Verification items for the finished model (mm, model axes). Face numbers are marked on the shaded views. A direction names the side the tool comes from. Give positions to 0.01 mm unless a question says otherwise; leave off trailing zeros. Write each loop counter-clockwise with the first axis right and the second up, starting at its lowest first coordinate (ties: lowest second). Pieces come first, ordered by that corner, then holes. Notation, with made-up numbers: (72.5, -17) -> (127.5, -17) arc R20 cw to (127.5, -8) -> close; hole circle Ø4 at (-6, -22.75). An arc over 180 degrees is marked (long way). Use CSV: the item, a comma, the result in double quotes. Start each with the question number.
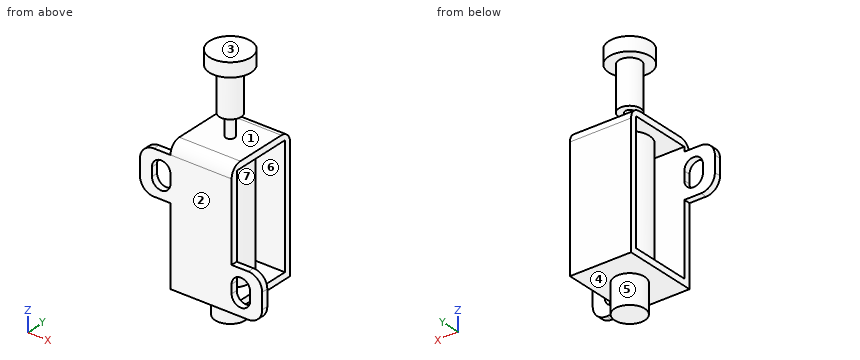
Autodesk Inventor part; units mm, degrees
ref_plane "Work Plane1" through (0, 8.5, 0) normal (0, 1, 0) x (1, 0, 0)
ref_plane "YZ Plane" through (0, 0, 0) normal (1, 0, 0) x (0, 1, 0)
ref_plane "XZ Plane" through (0, 0, 0) normal (0, 1, 0) x (-1, 0, 0)
sketch "Sketch1" plane through (0, 0, 0) normal (0, 1, 0) x (-1, 0, 0)
  line L0 (7, 15.2) -> (-7, 15.2)
  line L1 (-7, 15.2) -> (-7, -15.2)
  line L2 (-7, -15.2) -> (7, -15.2)
  line L3 (7, -15.2) -> (7, 15.2)
  point P0 (0, 0)
  dimension "d0" = 30.4
  dimension "d1" = 14
  dimension "d2" = 7
  dimension "d3" = 15.2
extrude "Extrusion1" add sketch "Sketch1" along normal blind 17
fillet "Fillet1" radius 2.54 2 edges at (0, 17, 15.2) (0, 0, 15.2)
sketch "Sketch2" plane through (7, 0, -15.2) normal (1, 0, 0) x (0, 0, -1)
  line L0 (-1.5, 15.5) -> (-28.9, 15.5)
  line L1 (-28.9, 15.5) -> (-28.9, 1.5)
  line L2 (-28.9, 1.5) -> (-1.5, 1.5)
  line L3 (-1.5, 1.5) -> (-1.5, 15.5)
  line L4 (-28.9, 8.5) -> (-30.4, 8.5) construction
  line L5 (-30.4, 2.54) -> (-30.4, 14.46)
  line L6 (-1.5, 9.1916) -> (0, 9.1916) construction
  line L7 (0, 0) -> (0, 17)
  line L8 (-13.3503, 1.5) -> (-13.3503, 0) construction
  line L9 (-15.2, 15.5) -> (-15.2, 17) construction
  line L10 (0, 17) -> (-27.86, 17)
  line L11 (-27.86, 0) -> (0, 0)
  point P0 (-15.2, 0)
  dimension "d7" = 1.5
extrude "Extrusion2" cut sketch "Sketch2" against normal blind 17
ref_plane "Work Plane1" through (0, 8.5, 0) normal (0, 1, 0) x (1, 0, 0)
sketch "Sketch4" plane through (0, 17, 0) normal (0, 1, 0) x (1, 0, 0)
  line L0 (7, 15.2) -> (-7, 15.2)
  line L1 (0, 15.2) -> (3.45, 15.2)
  line L2 (3.45, 15.2) -> (3.45, 21.8)
  line L3 (3.45, 21.8) -> (0, 21.8)
  line L4 (0, 21.8) -> (0, 15.2)
  line L5 (-7, -15.2) -> (7, -15.2)
  line L6 (0, 15.2) -> (4.5, 15.2)
  line L7 (4.5, 15.2) -> (4.5, -15.2)
  line L8 (4.5, -15.2) -> (0, -15.2)
  line L9 (0, -15.2) -> (0, 15.2)
  line L10 (1, -15.2) -> (0, -15.2)
  line L11 (0, -15.2) -> (0, -20.1)
  line L12 (0, -20.1) -> (1, -20.1)
  line L13 (1, -20.1) -> (1, -15.2)
  line L14 (0, -20.1) -> (2.5, -20.1)
  line L15 (2.5, -20.1) -> (2.5, -30.1)
  line L16 (2.5, -30.1) -> (0, -30.1)
  line L17 (0, -30.1) -> (0, -20.1)
  point P0 (0, 0)
  dimension "d10" = 3.45
  dimension "d11" = 51.9
  dimension "d12" = 10
  dimension "d14" = 4.9
  dimension "d15" = 2.5
  dimension "d16" = 1
  dimension "d17" = 4.5
sketch "Sketch5" plane through (0, 8.5, 0) normal (0, 1, 0) x (1, 0, 0)
  line L0 (0, 15.2) -> (3.45, 15.2)
  line L1 (3.45, 15.2) -> (3.45, 21.8)
  line L2 (3.45, 21.8) -> (0, 21.8)
  line L3 (0, 21.8) -> (0, 15.2)
  line L4 (0, 15.2) -> (4.5, 15.2)
  line L5 (4.5, 15.2) -> (4.5, -15.2)
  line L6 (4.5, -15.2) -> (0, -15.2)
  line L7 (0, -15.2) -> (0, 15.2)
  line L8 (1, -15.2) -> (0, -15.2)
  line L9 (0, -15.2) -> (0, -20.1)
  line L10 (0, -20.1) -> (1, -20.1)
  line L11 (1, -20.1) -> (1, -15.2)
  line L12 (0, -20.1) -> (2.5, -20.1)
  line L13 (2.5, -20.1) -> (2.5, -30.1)
  line L14 (2.5, -30.1) -> (0, -30.1)
  line L15 (0, -30.1) -> (0, -20.1)
  point P0 (0, 0)
  dimension "d18" = 3.45
  dimension "d19" = 51.9
  dimension "d20" = 10
  dimension "d21" = 4.9
  dimension "d22" = 2.5
  dimension "d23" = 1
  dimension "d24" = 4.5
revolve "Revolution1" add sketch "Sketch5" angle 360 about axis through (0, 8.5, 30.1) along (0, 0, -1)
sketch "Sketch6" plane through (0, 0, 0) normal (0, 1, 0) x (-1, 0, 0)
  line L0 (-7, -15.2) -> (7, -15.2)
  line L1 (-7, 12.66) -> (7, 12.66)
  line L2 (7, 12.66) -> (10.825, 12.66)
  line L3 (14, 9.485) -> (14, 5.835)
  line L4 (10.825, 2.66) -> (7, 2.66)
  line L5 (7, 2.66) -> (7, 12.66)
  line L6 (11.25, 6.66) -> (7, 6.66)
  line L7 (7, 6.66) -> (7, 8.66)
  line L8 (7, 8.66) -> (11.25, 8.66)
  line L9 (11.25, 8.66) -> (11.25, 6.66)
  line L10 (7, -15.2) -> (7, 12.66)
  line L11 (7, 7.66) -> (14, 7.66) construction
  circle A0 centre (9.125, 6.66) radius 2.125
  circle A1 centre (9.125, 8.66) radius 2.125
  arc A2 (10.825, 2.66) -> (14, 5.835) centre (10.825, 5.835) ccw
  arc A3 (14, 9.485) -> (10.825, 12.66) centre (10.825, 9.485) ccw
  line L12 (-1, 15.2) -> (1, 15.2)
  line L13 (7, -15.2) -> (7, 12.66)
  line L14 (7, 12.66) -> (7, -15.2)
  line L15 (7, -1.27) -> (-7, -1.27) construction
  line L16 (-7, -13.7) -> (-7, 13.7)
  line L17 (0, -1.27) -> (0, -15.2) construction
  line L18 (7, -15.2) -> (10.825, -15.2) construction
  line L19 (14, -12.025) -> (14, -8.375) construction
  line L20 (10.825, -5.2) -> (7, -5.2) construction
  line L21 (7, -5.2) -> (7, -15.2) construction
  line L22 (11.25, -9.2) -> (7, -9.2) construction
  line L23 (7, -9.2) -> (7, -11.2) construction
  line L24 (7, -11.2) -> (11.25, -11.2) construction
  line L25 (11.25, -11.2) -> (11.25, -9.2) construction
  line L26 (7, -10.2) -> (14, -10.2) construction
  circle A4 centre (9.125, -9.2) radius 2.125 construction
  circle A5 centre (9.125, -11.2) radius 2.125 construction
  arc A6 (14, -8.375) -> (10.825, -5.2) centre (10.825, -8.375) ccw construction
  arc A7 (10.825, -15.2) -> (14, -12.025) centre (10.825, -12.025) ccw construction
  line L27 (-7, -5.2) -> (-7, -15.2)
  line L28 (-7, -9.2) -> (-7, -11.2)
  line L29 (-7, -15.2) -> (-10.825, -15.2)
  line L30 (-7, -11.2) -> (-11.25, -11.2)
  line L31 (-11.25, -9.2) -> (-7, -9.2)
  line L32 (-11.25, -11.2) -> (-11.25, -9.2)
  circle A8 centre (-9.125, -11.2) radius 2.125
  circle A9 centre (-9.125, -9.2) radius 2.125
  arc A10 (-14, -12.025) -> (-10.825, -15.2) centre (-10.825, -12.025) ccw
  line L33 (-10.825, -5.2) -> (-7, -5.2)
  line L34 (-7, -10.2) -> (-14, -10.2) construction
  line L35 (-14, -12.025) -> (-14, -8.375)
  arc A11 (-10.825, -5.2) -> (-14, -8.375) centre (-10.825, -8.375) ccw
  point P0 (14, 2.66)
  point P1 (14, 12.66)
  point P2 (14, -5.2)
  point P3 (14, -15.2)
  point P4 (-14, -15.2)
  point P5 (-14, -5.2)
  dimension "d26" = 4.25
  dimension "d27" = 7
  dimension "d28" = 10
  dimension "d29" = 2
  dimension "d30" = 3.175
extrude "Extrusion3" add sketch "Sketch6" along normal blind 1.5 contours L29 A10 L35 A11 L33 L16 A9 L32 A8 L27 | L5 A0 L9 A1 L2 A3 L3 A2 L4
sketch "Sketch7" plane through (0, 8.5, 30.1) normal (0, 0, 1) x (1, 0, 0)
  circle A0 centre (0, 0) radius 2.5
  circle A1 centre (0, 0) radius 4.7625
  point P0 (0, -8.5)
  dimension "d33" = 9.525
extrude "Extrusion4" add sketch "Sketch7" along normal blind 3.175 contours A0 | A1
properties part number "Solenoid"
(1) Section check C-C on z = 17.5. Record the cut outline in (x, y).
(2) Draft check along Z on the marked faces 1, 2, 3 and 4. Enter one of: released by +Z, released by -Z, zero draft, split by the parting line, or undercut.
(3) Go/stop test with flat-tipped pins: pin 1 (0.8 mm diameter, centred on y = 0.5, z = -10.5, fed in from -X); pin 2 (0.8 mm diameter, centred on y = 1, z = 8, fed in from +X); pin 3 (5 mm diameter, centred on y = 10.5, z = 5, fed in from +X); pin 4 (1.5 mm diameter, centred on x = -9, y = 9, fed in from -Z). Record where each tip stops, or that it passes through.
(4) Thickness scan on line 1 (Z direction, x = 4.25, y = 6.5) (3 decimals); line 2 (Z direction, x = 2.5, y = 5) (3 decimals); line 3 (Y direction, x = -1.5, z = 0). Record the ranges inside material, lowest first. Write a range as from..to.
(5) Set-up check for the marked faces 5, 6 and 7: record each of +Z, -Z, +X, -X, +Y, -Y from which the full face is reachable in a straight line by a thin tool's end or side.
(6) Section check A-A on z = -3.5. Record the cut outline in (x, y), then the cut area to 3 significant figures.
(7) Section check B-B on x = 0. Give the number of separate pieces and of enclosed holes in the cut face, then the cut area to 3 significant figures.
Data:
1,outline,"circle Ø2 at (0, 8.5)"
2,face 1,"undercut"
2,face 2,"zero draft"
2,face 3,"released by +Z"
2,face 4,"released by -Z"
3,pin 1,"stops at x = -7"
3,pin 2,"stops at x = 7"
3,pin 3,"stops at x = 4.5"
3,pin 4,"passes through"
4,line 1,"z = -15.2..-13.7, 13.7..15.2, 30.1..33.275"
4,line 2,"z = -15.2..15.2, 30.1..33.275"
4,line 3,"y = 0..1.5, 4.26..12.74, 15.5..17"
5,face 5,"-Z"
5,face 6,"+X, -X"
5,face 7,"none"
6,outline,"(-7, 0) -> (7, 0) -> (7, 1.5) -> (-7, 1.5) -> close; (-7, 15.5) -> (7, 15.5) -> (7, 17) -> (-7, 17) -> close; circle Ø9 at (0, 8.5)"
6,area,"106 mm2"
7,separate pieces,"1"
7,enclosed holes,"2"
7,area,"513 mm2"
